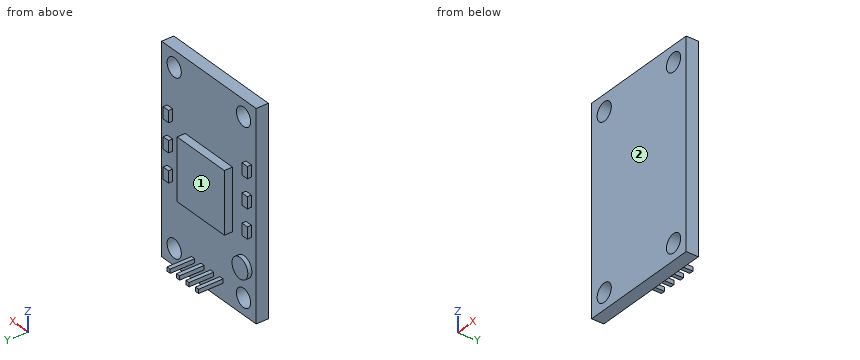
```python
from build123d import *

# Parameters (mm, degrees)
SKETCH1_W            = 30
SKETCH1_H            = 50
BOSS_EXTRUDE1_DEPTH  = 3
SKETCH2_R            = 2.25
CUT_EXTRUDE1_DEPTH   = 3
LPATTERN1_COUNT      = 2
LPATTERN1_PITCH      = 22
LPATTERN1_COUNT_DIR2 = 2
LPATTERN1_PITCH_DIR2 = 42
SKETCH3_W            = 1
SKETCH3_H            = 1
BOSS_EXTRUDE2_DEPTH  = 6
LPATTERN2_COUNT      = 4
LPATTERN2_PITCH      = 3
SKETCH4_W            = 15
SKETCH4_H            = 15
BOSS_EXTRUDE3_DEPTH  = 2
SKETCH5_W            = 1.709574014
SKETCH5_H            = 2.849290021
BOSS_EXTRUDE4_DEPTH  = 1
LPATTERN3_COUNT      = 3
LPATTERN3_PITCH      = 7
LPATTERN3_COUNT_DIR2 = 2
LPATTERN3_PITCH_DIR2 = 25
SKETCH6_R            = 2.5
BOSS_EXTRUDE5_DEPTH  = 1


with BuildPart() as part:
    # Sketch1 → Boss-Extrude1 (new body)
    with BuildSketch(Plane(origin=(0, 0, 0), x_dir=(1, 0, 0), z_dir=(0, 1, 0))):
        Rectangle(SKETCH1_W, SKETCH1_H)
    extrude(amount=BOSS_EXTRUDE1_DEPTH)

    # Sketch2 → Cut-Extrude1 (cut)
    with BuildSketch(Plane(origin=(0, 3, 0), x_dir=(1, 0, 0), z_dir=(0, 1, 0))):
        with Locations(Location((-11, 21, 0), (0, 0, 270))):
            Circle(SKETCH2_R)
    cut_extrude1 = extrude(amount=-CUT_EXTRUDE1_DEPTH, mode=Mode.SUBTRACT)

    # LPattern1: Cut-Extrude1 2 × 2
    with Locations(*[(i * LPATTERN1_PITCH, 0, j * LPATTERN1_PITCH_DIR2) for i in range(LPATTERN1_COUNT) for j in range(LPATTERN1_COUNT_DIR2) if (i, j) != (0, 0)]):
        add(cut_extrude1, mode=Mode.SUBTRACT)

    # Sketch3 → Boss-Extrude2 (add)
    with BuildSketch(Plane(origin=(0, 3, 0), x_dir=(1, 0, 0), z_dir=(0, 1, 0))):
        with Locations((-4, 20.5)):
            Rectangle(SKETCH3_W, SKETCH3_H)
    boss_extrude2 = extrude(amount=BOSS_EXTRUDE2_DEPTH)

    # LPattern2: Boss-Extrude2 ×4
    with Locations(*[(i * LPATTERN2_PITCH, 0, 0) for i in range(1, LPATTERN2_COUNT)]):
        add(boss_extrude2)

    # Sketch4 → Boss-Extrude3 (add)
    with BuildSketch(Plane(origin=(0, 3, 0), x_dir=(1, 0, 0), z_dir=(0, 1, 0))):
        Rectangle(SKETCH4_W, SKETCH4_H)
    extrude(amount=BOSS_EXTRUDE3_DEPTH)

    # Sketch5 → Boss-Extrude4 (add)
    with BuildSketch(Plane(origin=(0, 3, 0), x_dir=(1, 0, 0), z_dir=(0, 1, 0))):
        with Locations((-12.643724472, -9.7232022)):
            Rectangle(SKETCH5_W, SKETCH5_H)
    boss_extrude4 = extrude(amount=BOSS_EXTRUDE4_DEPTH)

    # LPattern3: Boss-Extrude4 3 × 2
    with Locations(*[(j * LPATTERN3_PITCH_DIR2, 0, -i * LPATTERN3_PITCH) for i in range(LPATTERN3_COUNT) for j in range(LPATTERN3_COUNT_DIR2) if (i, j) != (0, 0)]):
        add(boss_extrude4)

    # Sketch6 → Boss-Extrude5 (add)
    with BuildSketch(Plane(origin=(0, 3, 0), x_dir=(1, 0, 0), z_dir=(0, 1, 0))):
        with Locations(Location((-11.14784721, 13.64097598, 0), (0, 0, 90))):
            Circle(SKETCH6_R)
    extrude(amount=BOSS_EXTRUDE5_DEPTH)


solid = part.part
```
Could you check a few things on this model? Use its own coordinates, in mm. Face numbers are marked on the shaded views. A direction names the side the tool comes from. Coordinates: 2 decimals unless noted, no trailing zeros. Loops run counter-clockwise (first coordinate to the right, second up) from the corner with the lowest first, then second, coordinate; pieces in that order, holes last. Notation, with made-up numbers: M 61.25,16 L 69.25,16 A35 ccw 69.25,52 Z; hole C -3.75,-32.75 d3. An arc over 180 degrees is marked long. Put each result on its own line as item: value. Start each with the question number.
(1) Suppose I cut it at A-A on y = 2. Please give me the cut outline in (x, z), then the cut area to 3 significant figures.
(2) Suppose I cut it at B-B on x = 11. Please give me the cut outline in (y, z).
(3) Will these pins go through, and if not, where does the flat tip stop? P1, Ø1, axis at x = 12, z = -11.5, coming from the +Y side; P2, Ø0.8, axis at y = 3.5, z = -4.5, coming from the -X side; P3, Ø0.8, axis at x = 5, y = 6.5, coming from the +Z side.
(4) I need wall thicknesses on line 1 (X direction, y = 1.9, z = 21); line 2 (Y direction, x = 12.5, z = 7); line 3 (Z direction, x = -4, y = 7.75). Which ranges of each line are inside material? Lowest first, please. Write a range as from..to.
(5) For the marked faces 1 and 2, which set-ups out of +Z, -Z, +X, -X, +Y, -Y let a thin tool reach every point of the face, with its end or its side?
(6) Suppose I cut it at D-D on y = 5.5. Please give me the cut outline in (x, z), then the cut area to 3 significant figures.
(7) Suppose I cut it at C-C on z = 21. Please give me the cut outline in (x, y).
Solutions:
1. outline: M -15,-25 L 15,-25 L 15,25 L -15,25 Z; hole C -11,-21 d4.5; hole C -11,21 d4.5; hole C 11,-21 d4.5; hole C 11,21 d4.5
1. area: 1,440 mm2
2. outline: M 0,-25 L 3,-25 L 3,-23.25 L 0,-23.25 Z; M 0,-18.75 L 3,-18.75 L 3,18.75 L 0,18.75 Z; M 0,23.25 L 3,23.25 L 3,25 L 0,25 Z
3. P1: stops at y = 3
3. P2: stops at x = -13.5
3. P3: stops at z = -20
4. line 1: x = -15..-13.25, -8.75..8.75, 13.25..15
4. line 2: y = 0..3
4. line 3: z = -21..-20
5. face 1: +Z, +X, -X, +Y
5. face 2: +Z, -Z, +X, -X, -Y
6. outline: M -4.5,-21 L -3.5,-21 L -3.5,-20 L -4.5,-20 Z; M -1.5,-21 L -0.5,-21 L -0.5,-20 L -1.5,-20 Z; M 1.5,-21 L 2.5,-21 L 2.5,-20 L 1.5,-20 Z; M 4.5,-21 L 5.5,-21 L 5.5,-20 L 4.5,-20 Z
6. area: 4.00 mm2
7. outline: M -15,0 L -13.25,0 L -13.25,3 L -15,3 Z; M -8.75,0 L 8.75,0 L 8.75,3 L -8.75,3 Z; M 13.25,0 L 15,0 L 15,3 L 13.25,3 Z
